from build123d import *

# Parameters (mm, degrees)
F0_W     = 209.3077600002
F0_H     = 131.40617311
F0_W_2   = 189.4957572222
F0_H_2   = 111.594170332
F1_DEPTH = 117.856
F2_W     = 76.2
F2_H     = 9.906001389
F3_DEPTH = 38.1
F4_R     = 12.7
F5_DEPTH = 209.3087600002


with BuildPart() as f1:
    # F0 (on Top) → F1 (new body)
    with BuildSketch(Plane.XY):
        Rectangle(F0_W, F0_H)
        Rectangle(F0_W_2, F0_H_2, mode=Mode.SUBTRACT)
    extrude(amount=F1_DEPTH)

    # F2 (on face) → F3 (cut)
    with BuildSketch(Plane.XY.offset(117.856)):
        with Locations((0, 60.7500858605)):
            Rectangle(F2_W, F2_H)
        with Locations((0, -60.7500858605)):
            Rectangle(F2_W, F2_H)
    extrude(amount=-F3_DEPTH, mode=Mode.SUBTRACT)

    # F4 (on face) → F5 (cut, through all)
    with BuildSketch(Plane.YZ.offset(104.6538800001)):
        with Locations((0, 58.928)):
            Circle(F4_R)
    extrude(amount=-F5_DEPTH, mode=Mode.SUBTRACT)


solid = f1.part
Here's how the part is built. I have some questions about the finished solid (model axes, mm). A direction names the side the tool comes from. Coordinates: 2 decimals unless noted, no trailing zeros. Order: outer loops, then holes, each group sorted by start corner. A loop starts at its lowest first (then second) coordinate and runs counter-clockwise, first axis right, second up.
Item 1: For faces 4 (the face through (-104.654, -1, 45)), 5 (the face through (94.748, -13, 58)), 6 (the face through (-38.1, -61, 99)), which set-ups out of +Z, -Z, +X, -X, +Y, -Y let a thin tool reach every point of the face, with its end or its side?
Result sheet:
face 4: +Z, -Z, -X, +Y, -Y
face 5: +Z, -Z
face 6: +Z, +Y, -Y
Item 2: If we mould it in two halves opening along Y, with no side actions, what happens to faces 1 (the face through (38.1, 61, 99)), 2 (the face through (-1, -65.703, 58)), 3 (the face through (-1, -55.797, 58))? For each: +Y half, -Y half, draft (parallel to the pull), parting line (faces both ways), or undercut.
Result sheet:
face 1: draft
face 2: -Y half
face 3: undercut
Item 3: If we section it at C-C on x = -29.5: List the corners of the cut face in (y, z) for me, plus the area to 3 significant figures.
Result sheet:
outline: (-65.7, 0) - (-55.8, 0) - (-55.8, 79.76) - (-65.7, 79.76) - close; (55.8, 0) - (65.7, 0) - (65.7, 79.76) - (55.8, 79.76) - close
area: 1,580 mm2
Item 4: For P1, Ø23, axis at y = 0, z = 58.928, coming from the +X side; P2, Ø11, axis at x = 6.5, y = -61.5, coming from the +Z side, each with a flat end and sliding along its axis, tell me the tip position at first contact or that it passes through.
Result sheet:
P1: passes through
P2: stops at z = 79.76
Item 5: I need wall thicknesses on line 1 (Y direction, x = 64, z = 71); line 2 (X direction, y = 40.5, z = 16); line 3 (Z direction, x = -101.25, y = 0). Which ranges of each line are inside material? Lowest first, please.
Result sheet:
line 1: y = -65.7 to -55.8, 55.8 to 65.7
line 2: x = -104.65 to -94.75, 94.75 to 104.65
line 3: z = 0 to 46.23, 71.63 to 117.86
Item 6: If we section it at A-A on y = 23.5: List the corners of the cut face in (x, z) for me, plus the area to 3 significant figures.
Result sheet:
outline: (-104.65, 0) - (-94.75, 0) - (-94.75, 117.86) - (-104.65, 117.86) - close; (94.75, 0) - (104.65, 0) - (104.65, 117.86) - (94.75, 117.86) - close
area: 2,330 mm2
Item 7: If we section it at B-B on z = 95.5: List the corners of the cut face in (x, y) for me, plus the area to 3 significant figures.
Result sheet:
outline: (-104.65, -65.7) - (-38.1, -65.7) - (-38.1, -55.8) - (-94.75, -55.8) - (-94.75, 55.8) - (-38.1, 55.8) - (-38.1, 65.7) - (-104.65, 65.7) - close; (38.1, -65.7) - (104.65, -65.7) - (104.65, 65.7) - (38.1, 65.7) - (38.1, 55.8) - (94.75, 55.8) - (94.75, -55.8) - (38.1, -55.8) - close
area: 4,850 mm2
Item 8: If we section it at D-D on y = 0: List the corners of the cut face in (x, z) for me.
Result sheet:
outline: (-104.65, 0) - (-94.75, 0) - (-94.75, 46.23) - (-104.65, 46.23) - close; (-104.65, 71.63) - (-94.75, 71.63) - (-94.75, 117.86) - (-104.65, 117.86) - close; (94.75, 0) - (104.65, 0) - (104.65, 46.23) - (94.75, 46.23) - close; (94.75, 71.63) - (104.65, 71.63) - (104.65, 117.86) - (94.75, 117.86) - close
